Check sheet for the drawn part. Datum: minimum x, y, z corner. Units: mm. Round coordinates to 2 decimals unless told otherwise and drop trailing zeros. Loops run counter-clockwise (first coordinate to the right, second up) from the corner with the lowest first, then second, coordinate; pieces in that order, holes last. Notation, with made-up numbers: (9.25, -20.75) -> (49.25, -20.75) arc R8 cw to (49.25, -16.75) -> close; hole circle Ø5 at (88, 13). An arc over 180 degrees is marked (long way). Use CSV: the item, a comma, the result in double quotes. Start each with the question number.
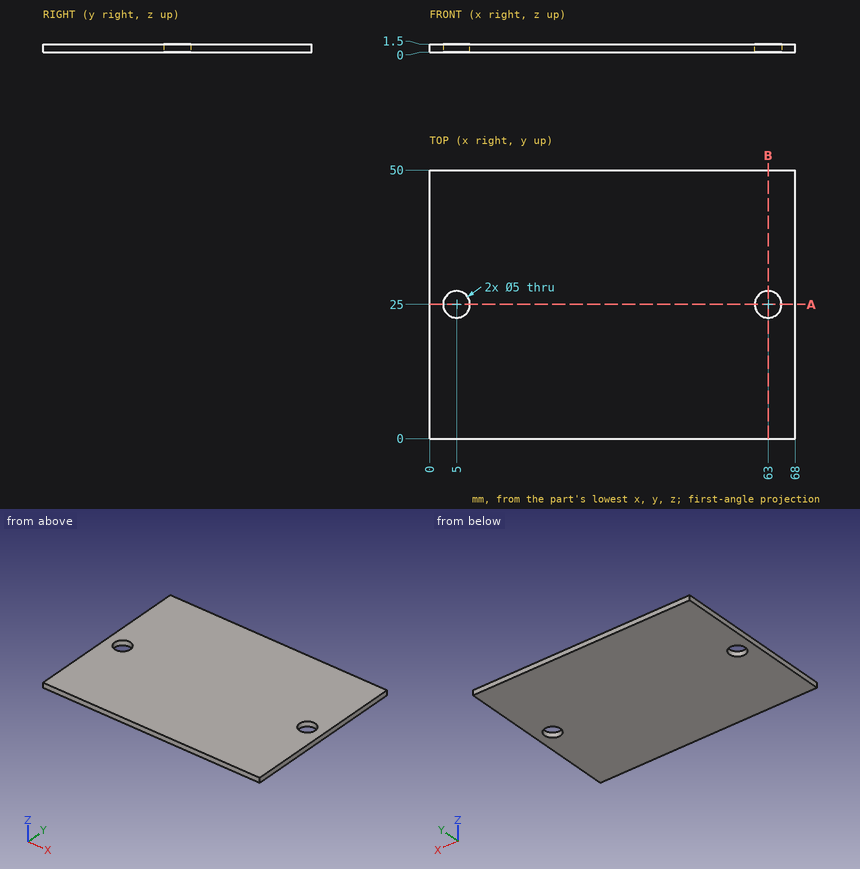
Q1. Cross-section at A-A (y = 25). Record the boundary of the cut face in (x, z), and give its area (3 significant figures).
Q2. Depth check by flat-ended pin: pin 1 Ø12 at (x, y) = (17.5, 27.5) entering from -Z; pin 2 Ø4.5 at (x, y) = (63, 25) entering from -Z. Enter the tip coordinate at first touch or a pass-through.
Q3. Cross-section at B-B (x = 63). Record the boundary of the cut face in (y, z).
Q4. Thickness scan on L1, parallel to Y at x = 63, z = 0.6; L2, parallel to Y at x = 62.5, z = 1.2. Record the ranges inside material, lowest first. Write a range as from..to.
Answer list:
1,outline,"(0, 0) -> (2.5, 0) -> (2.5, 1.5) -> (0, 1.5) -> close; (7.5, 0) -> (60.5, 0) -> (60.5, 1.5) -> (7.5, 1.5) -> close; (65.5, 0) -> (68, 0) -> (68, 1.5) -> (65.5, 1.5) -> close"
1,area,"87.0 mm2"
2,pin 1,"stops at z = 0"
2,pin 2,"passes through"
3,outline,"(0, 0) -> (22.5, 0) -> (22.5, 1.5) -> (0, 1.5) -> close; (27.5, 0) -> (50, 0) -> (50, 1.5) -> (27.5, 1.5) -> close"
4,L1,"y = 0..22.5, 27.5..50"
4,L2,"y = 0..22.55, 27.45..50"
